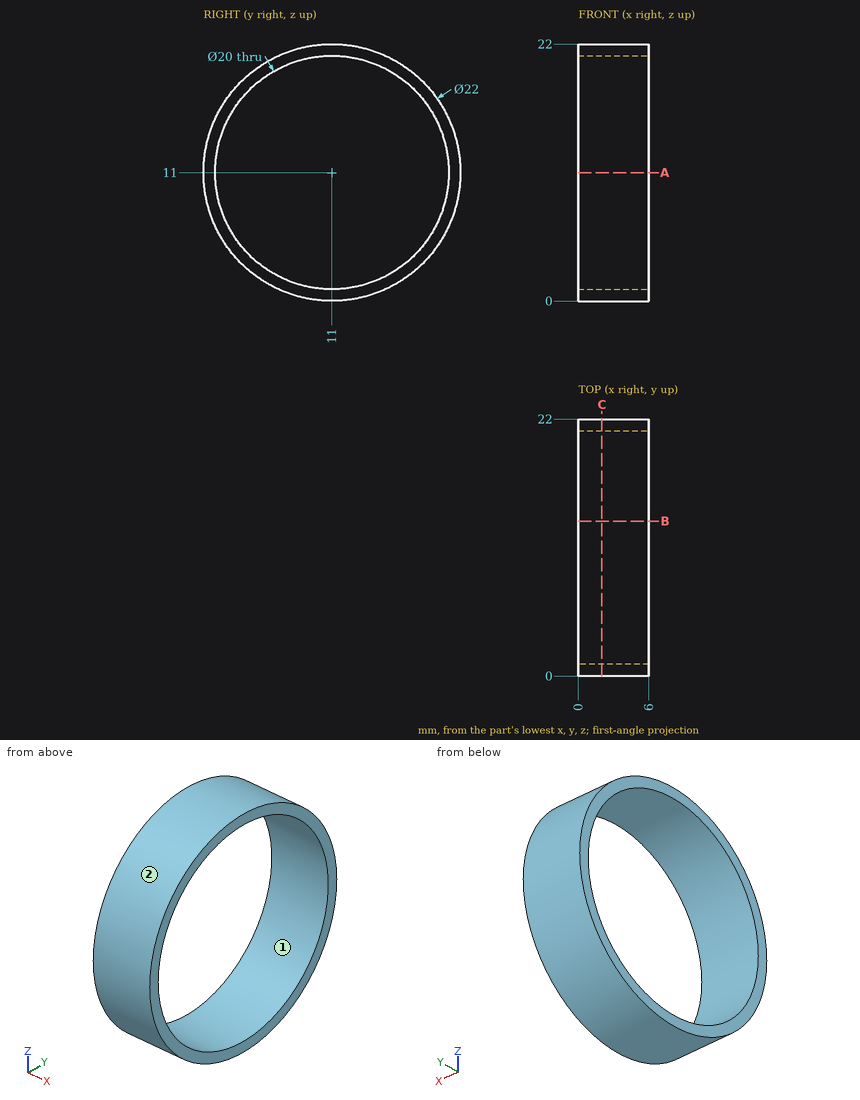
Geometry: see drawing. Coordinates: mm, zero at the bounding-box minimum. Give positions to 0.01 mm unless a question says otherwise; leave off trailing zeros. Order: outer loops, then holes, each group sorted by start corner. A loop starts at its lowest first (then second) coordinate and runs counter-clockwise, first axis right, second up. Notation, with made-up numbers: (81, 32.25) -> (139, 32.25) arc R21 cw to (139, 43.25) -> close; hole circle Ø1 at (4, 10). An arc over 180 degrees is marked (long way). Write item = value, one per line.
Q1. Pull-direction query (Z, two-part tool) for the marked faces 1 and 2; classes: released by +Z, released by -Z, zero draft, split by the parting line, or undercut.
Data:
face_1 = undercut
face_2 = split by the parting line
Q2. Material intervals for line 1 (Z direction, x = 3.8, y = 11); line 2 (Z direction, x = 1.8, y = 13.5); line 3 (Y direction, x = 2, z = 14.75), sorted ascending. Write a range as from..to.
Data:
line_1 = 0..1, 21..22
line_2 = 0.29..1.32, 20.68..21.71
line_3 = 0.66..1.73, 20.27..21.34
Q3. Cut plane A-A, the plane z = 11. Output: boundary loops of the cut face in (x, y), and give its area (3 significant figures).
Data:
outline = (0, 0) -> (6, 0) -> (6, 1) -> (0, 1) -> close; (0, 21) -> (6, 21) -> (6, 22) -> (0, 22) -> close
area = 12.0 mm^2
Q4. Pin query (flat end, axial travel): pin 1 (1.5 mm diameter, centred on y = 11, z = 19, fed in from +X); pin 2 (6 mm diameter, centred on y = 19, z = 18, fed in from -X); pin 3 (2 mm diameter, centred on x = 3, y = 13, fed in from -Z). Return the tip coordinate at first contact, or that it passes through.
Data:
pin_1 = through
pin_2 = 0
pin_3 = 0.05
Q5. Cut plane C-C, the plane x = 2. Output: boundary loops of the cut face in (y, z), and give its area (3 significant figures).
Data:
outline = circle Ø22 at (11, 11); hole circle Ø20 at (11, 11)
area = 66.0 mm^2
Q6. Cut plane B-B, the plane y = 13.25. Output: boundary loops of the cut face in (x, z), and give its area (3 significant figures).
Data:
outline = (0, 0.23) -> (6, 0.23) -> (6, 1.26) -> (0, 1.26) -> close; (0, 20.74) -> (6, 20.74) -> (6, 21.77) -> (0, 21.77) -> close
area = 12.3 mm^2
